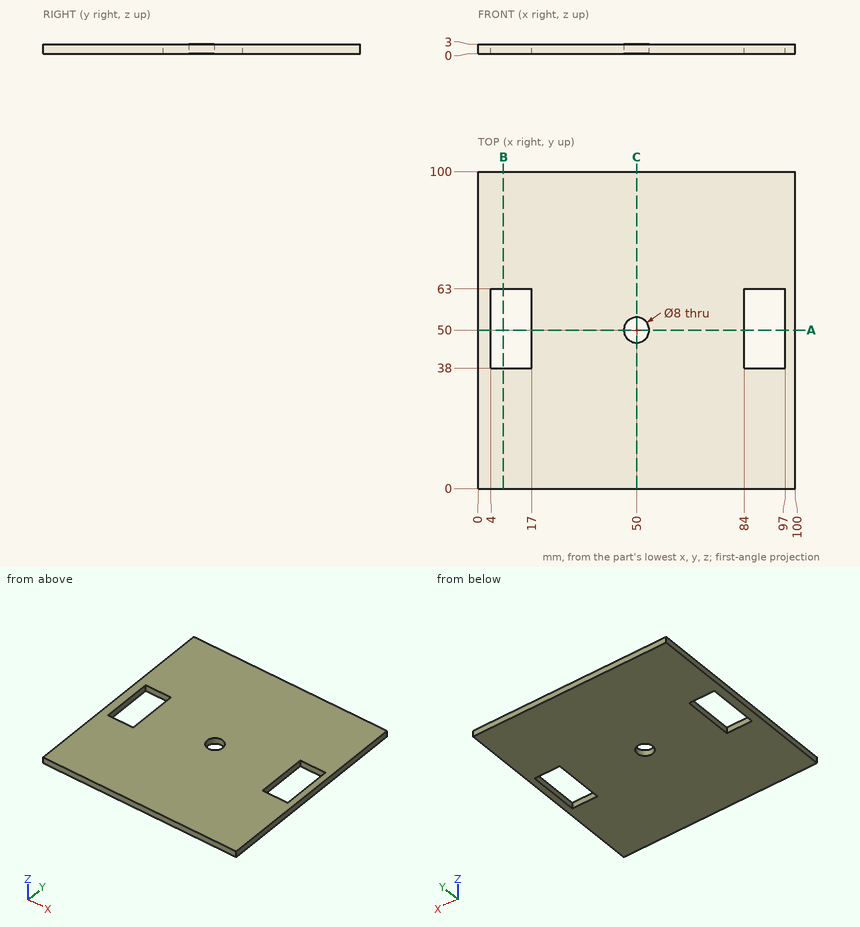
Part print with two shaded views. Sizes in mm from the minimum x, y, z corner. Coordinates: 2 decimals unless noted, no trailing zeros. Loops run counter-clockwise (first coordinate to the right, second up) from the corner with the lowest first, then second, coordinate; pieces in that order, holes last. Notation, with made-up numbers: M 57,17 L 75,17 A22 cw 75,38 Z; hole C 6,30 d1. An arc over 180 degrees is marked long. Use CSV: the item, a comma, the result in double quotes. Start each with the question number.
1. Band-saw the part on C-C, the plane x = 50. List the corners of the cut face in (y, z).
2. Band-saw the part on A-A, the plane y = 50. List the corners of the cut face in (x, z).
3. Probe probe 1 along X at (y, z) = (55.5, 2.35); probe 2 along Y at (x, z) = (88, 1.9); probe 3 along Y at (x, z) = (50, 1.8). List the from-to ranges inside material, lowest first. Write a range as [from, to].
4. Band-saw the part on B-B, the plane x = 8. List the corners of the cut face in (y, z), then the cut area to 3 significant figures.
Entries:
1,outline,"M 0,0 L 46,0 L 46,3 L 0,3 Z; M 54,0 L 100,0 L 100,3 L 54,3 Z"
2,outline,"M 0,0 L 4,0 L 4,3 L 0,3 Z; M 17,0 L 46,0 L 46,3 L 17,3 Z; M 54,0 L 84,0 L 84,3 L 54,3 Z; M 97,0 L 100,0 L 100,3 L 97,3 Z"
3,probe 1,"x = [0, 4], [17, 84], [97, 100]"
3,probe 2,"y = [0, 38], [63, 100]"
3,probe 3,"y = [0, 46], [54, 100]"
4,outline,"M 0,0 L 38,0 L 38,3 L 0,3 Z; M 63,0 L 100,0 L 100,3 L 63,3 Z"
4,area,"225 mm2"
